Part model, mm, in its own coordinate system. A direction names the side the tool comes from. Coordinates: 2 decimals unless noted, no trailing zeros. Loops run counter-clockwise (first coordinate to the right, second up) from the corner with the lowest first, then second, coordinate; pieces in that order, holes last. Notation, with made-up numbers: (65, -39.75) - (108, -39.75) arc R18 cw to (108, -4.75) - close; hole circle Ø9 at (-39, 31.5). An arc over 180 degrees is marked (long way). Use a Markdown table: item, result. Add a question column.
1) Band-saw the part on C-C (y = 25). Give the cut face in (x, z).
2) Band-saw the part on A-A (y = 65). Give the cut face in (x, z), plus the area to 3 significant figures.
3) Band-saw the part on B-B (x = 10). Give the number of separate pieces and of enclosed holes in the cut face, plus the area to 3 significant figures.
4) Drop flat-ended pins along their axis: P1, Ø2, axis at x = 15, y = 42, coming from the -Z side; P2, Ø3.5, axis at x = 12.5, y = 67.5, coming from the +Z side; P3, Ø2.5, axis at x = 10.5, y = 83.5, coming from the -Z side. Give the stop position or say it passes through.
5) Probe probe 1 along Y at (x, z) = (10, 3.1); probe 2 along Y at (x, z) = (10, 9.9); probe 3 along X at (y, z) = (85, 3.6). List the from-to ranges inside material, lowest first. Write a range as [from, to].
6) Pull direction X, two halves, no side cores. Call faces 6 (the face through (20, 49, 9)), 7 (the face through (13, 85, 4.15)), 8 (the face through (10, 100, 9)), 9 (the face through (0, 49, 9)): +X half, -X half, draft (parallel to the pull), parting line (faces both ways), or undercut.
7) Tool access for faces 1 (the face through (14.16, 66.72, 2.89)), 2 (the face through (12.62, 84.17, 8.02)), 3 (the face through (7, 84, 12)), 4 (the face through (10, 10, 5)), 5 (the face through (9.856, 5.07, 2.087)): list every direction of +Z, -Z, +X, -X, +Y, -Y with a clear straight run to the whole face (end or side of a thin tool).
from build123d import *

# Parameters (mm, degrees)
BOX_W           = 20
BOX_H           = 100
BOX_DEPTH       = 20
SKETCH007_R     = 2.75
POCKET003_DEPTH = 20
SKETCH009_R     = 4.5
POCKET004_DEPTH = 4.15
SKETCH008_R     = 25
POCKET005_DEPTH = 100.001
SKETCH_W        = 30
SKETCH_H        = 20
POCKET_DEPTH    = 20.001
SKETCH010_R     = 2.1
POCKET006_DEPTH = 20.001
SKETCH011_R     = 5.5
POCKET007_DEPTH = 8
FILLET_R        = 1.5


with BuildPart() as part:
    # Box → Box (new body)
    with BuildSketch(Plane(origin=(-10, 0, -8), x_dir=(1, 0, 0), z_dir=(0, 0, 1))):
        with Locations((10, 50)):
            Rectangle(BOX_W, BOX_H)
    extrude(amount=BOX_DEPTH)

    # Sketch007 (on Face5 of Box) → Pocket003 (cut)
    with BuildSketch(Plane(origin=(-10, 0, -8), x_dir=(1, 0, 0), z_dir=(0, 0, -1))):
        with Locations((10, -65)):
            Circle(SKETCH007_R)
        with Locations((10, -85)):
            Circle(SKETCH007_R)
    extrude(amount=-POCKET003_DEPTH, mode=Mode.SUBTRACT)

    # Sketch009 (on Face5 of Pocket003) → Pocket004 (cut)
    with BuildSketch(Plane(origin=(-10, 0, -8), x_dir=(1, 0, 0), z_dir=(0, 0, -1))):
        with Locations((10, -85)):
            Circle(SKETCH009_R)
        with Locations((10, -65)):
            Circle(SKETCH009_R)
    extrude(amount=-POCKET004_DEPTH, mode=Mode.SUBTRACT)

    # Sketch008 (on Face4 of Pocket004) → Pocket005 (cut, through all)
    with BuildSketch(Plane(origin=(-10, 100, -8), x_dir=(-1, 0, 0), z_dir=(0, 1, 0))):
        with Locations((-10, -22.912878)):
            Circle(SKETCH008_R)
    extrude(amount=-POCKET005_DEPTH, mode=Mode.SUBTRACT)


with BuildPart() as part_1:
    # BaseFeature placement: moved
    add(part.part.moved(Location((10, 0, 8))))

    # Sketch (on Face1 of BaseFeature) → Pocket (cut, through all)
    with BuildSketch(Plane(origin=(0, 0, 0), x_dir=(0, -1, 0), z_dir=(-1, 0, 0))):
        with Locations((-25, -2)):
            Rectangle(SKETCH_W, SKETCH_H)
    extrude(amount=-POCKET_DEPTH, mode=Mode.SUBTRACT)

    # Sketch010 (on Face2 of Pocket) → Pocket006 (cut, through all)
    with BuildSketch(Plane.XY.offset(20)):
        with Locations((10, 25)):
            Circle(SKETCH010_R)
    extrude(amount=-POCKET006_DEPTH, mode=Mode.SUBTRACT)

    # Sketch011 (on Face2 of Pocket006) → Pocket007 (cut)
    with BuildSketch(Plane.XY.offset(20)):
        with Locations((10, 85)):
            Circle(SKETCH011_R)
        with Locations((10, 65)):
            Circle(SKETCH011_R)
    extrude(amount=-POCKET007_DEPTH, mode=Mode.SUBTRACT)

    # Sphere → Sphere (revolve, cut)
    with BuildSketch(Plane(origin=(10, 25, 26), x_dir=(1, 0, 0), z_dir=(0, -1, 0))):
        with BuildLine():
            ThreePointArc((0, -15), (15, 0), (0, 15))
            Line((0, 15), (0, -15))
        make_face()
    revolve(axis=Axis((10, 25, 26), (0, 0, 1)), mode=Mode.SUBTRACT)

    # Fillet
    fillet_edges = [part_1.edges().sort_by_distance(p)[0] for p in [
        (20, 67.216991, 20),
        (0, 67.216991, 20),
        (10, 100, 20),
        (0, 7.783009, 20),
        (20, 7.783009, 20),
        (10, 0, 20),
        (0, 0, 10),
        (0, 100, 10),
        (20, 100, 10),
        (20, 0, 10),
        (4.5, 65, 20),
        (4.5, 85, 20),
    ]]
    fillet(fillet_edges, radius=FILLET_R)


solid = part_1.part
Answer block:
| question | item | result |
|---|---|---|
| 1 | outline | (0, 8) - (7.9, 8) - (7.9, 11.15) arc R15 cw to (0, 14.82) - close; (12.1, 8) - (20, 8) - (20, 14.82) arc R15 cw to (12.1, 11.15) - close |
| 2 | outline | (0, 0) arc R25 cw to (5.5, 1.68) - (5.5, 4.15) - (7.25, 4.15) - (7.25, 12) - (4.5, 12) - (4.5, 18.5) arc R1.5 ccw to (3, 20) - (1.5, 20) arc R1.5 ccw to (0, 18.5) - close; (12.75, 4.15) - (14.5, 4.15) - (14.5, 1.68) arc R25 cw to (20, 0) - (20, 18.5) arc R1.5 ccw to (18.5, 20) - (17, 20) arc R1.5 ccw to (15.5, 18.5) - (15.5, 12) - (12.75, 12) - close |
| 2 | area | 219 mm2 |
| 3 | separate pieces | 4 |
| 3 | enclosed holes | 0 |
| 3 | area | 1,120 mm2 |
| 4 | P1 | z = 1.36 |
| 4 | P2 | z = 12 |
| 4 | P3 | z = 4.15 |
| 5 | probe 1 | [0, 10], [40, 60.5], [69.5, 80.5], [89.5, 100] |
| 5 | probe 2 | [0, 22.9], [27.1, 62.25], [67.75, 82.25], [87.75, 100] |
| 5 | probe 3 | [0, 5.5], [14.5, 20] |
| 6 | face 6 | +X half |
| 6 | face 7 | undercut |
| 6 | face 8 | draft |
| 6 | face 9 | -X half |
| 7 | face 1 | -Z |
| 7 | face 2 | +Z, -Z |
| 7 | face 3 | +Z |
| 7 | face 4 | -Z, +X, -X |
| 7 | face 5 | -Z, +Y, -Y |
